The figure shows three views and two pictorial views of one solid part (mm, origin at its lowest corner). Answer the questions. Round coordinates to 2 decimals unless told otherwise and drop trailing zeros. Loops run counter-clockwise (first coordinate to the right, second up) from the corner with the lowest first, then second, coordinate; pieces in that order, holes last. Notation, with made-up numbers: (6, 66) -> (23, 66) arc R31 cw to (23, 101) -> close; hole circle Ø7 at (-36, 63). An arc over 180 degrees is marked (long way). Put each result on its own line as item: value.
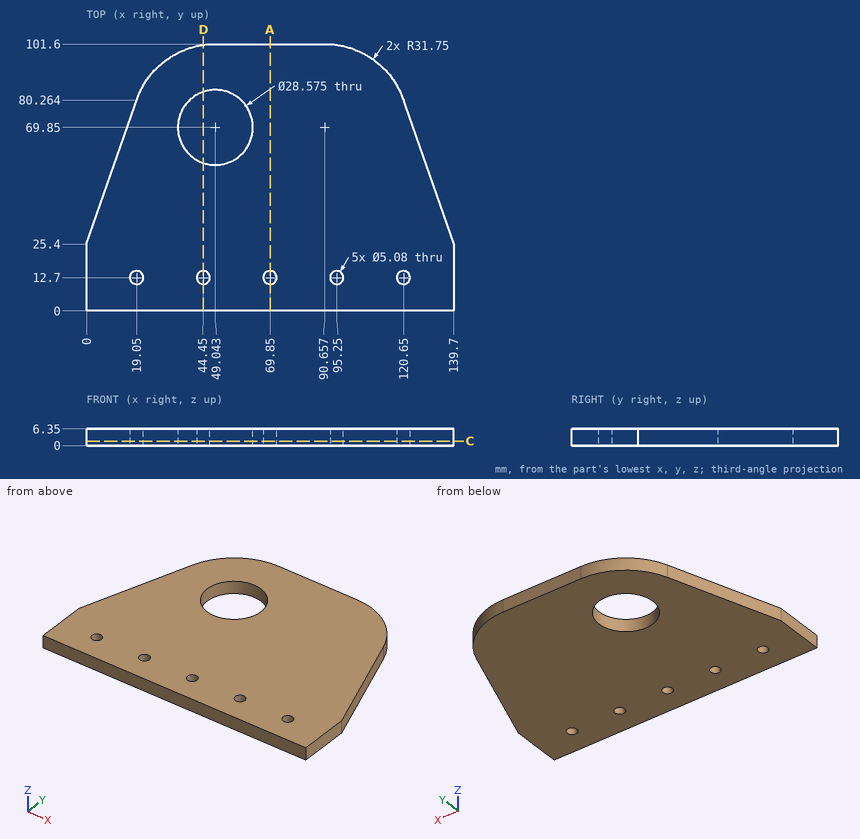
Item 1: The part is cut by section D-D (x = 44.45). Determine the outline of the cut face in (y, z), then the cut area to 3 significant figures.
Derived:
outline: (0, 0) -> (10.16, 0) -> (10.16, 6.35) -> (0, 6.35) -> close; (15.24, 0) -> (56.32, 0) -> (56.32, 6.35) -> (15.24, 6.35) -> close; (83.38, 0) -> (101.27, 0) -> (101.27, 6.35) -> (83.38, 6.35) -> close
area: 439 mm^2
Item 2: The part is cut by section A-A (x = 69.85). Determine the outline of the cut face in (y, z).
Derived:
outline: (0, 0) -> (10.16, 0) -> (10.16, 6.35) -> (0, 6.35) -> close; (15.24, 0) -> (101.6, 0) -> (101.6, 6.35) -> (15.24, 6.35) -> close
Item 3: The part is cut by section C-C (z = 1.75). State how many separate pieces and enclosed holes the cut face has, then the cut area to 3 significant figures.
Derived:
separate pieces: 1
enclosed holes: 6
area: 11,200 mm^2
Item 4: Find the intervals of material crossed by line 1 along X through (y, z) = (14, 1.75); line 2 along Y through (x, z) = (69.85, 4.5); line 3 along Y through (x, z) = (44.45, 1.75) (1 decimal), in increasing order.
Derived:
line 1: x = 0 to 16.87, 21.23 to 42.27, 46.63 to 67.67, 72.03 to 93.07, 97.43 to 118.47, 122.83 to 139.7
line 2: y = 0 to 10.16, 15.24 to 101.6
line 3: y = 0 to 10.2, 15.2 to 56.3, 83.4 to 101.3
Item 5: Flat-ended cylindrical pins translate along their axes: pin 1 Ø3 at (y, z) = (82.5, 3) entering from +X (1 decimal); pin 2 Ø4.5 at (x, y) = (120.65, 12.7) entering from -Z; pin 3 Ø1 at (y, z) = (30.5, 4) entering from -X. Find the tip coordinate at first contact, or state that the pin passes through.
Derived:
pin 1: stops at x = 120.4
pin 2: passes through
pin 3: stops at x = 1.6
